Work out the finished part from the listing and answer in its coordinate system (mm). Face numbers are marked on the shaded views. A direction names the side the tool comes from. Round coordinates to 2 decimals unless told otherwise and drop trailing zeros. Loops run counter-clockwise (first coordinate to the right, second up) from the corner with the lowest first, then second, coordinate; pieces in that order, holes last. Notation, with made-up numbers: M -15.75,9.25 L 2.25,9.25 A25 ccw 2.25,25.25 Z; hole C 35.5,28 d8. An arc over 180 degrees is marked long. One line per item, written item: value.
Autodesk Inventor part; units mm, degrees
ref_plane "YZ Plane" through (0, 0, 0) normal (1, 0, 0) x (0, 1, 0)
ref_plane "XZ Plane" through (0, 0, 0) normal (0, 1, 0) x (-1, 0, 0)
ref_plane "XY Plane" through (0, 0, 0) normal (0, 0, 1) x (1, 0, 0)
sketch "Sketch1" plane through (0, 0, 0) normal (0, 1, 0) x (-1, 0, 0)
  line L0 (0, 0) -> (-127, 0)
  line L1 (-127, 0) -> (-127, -124.46)
  line L2 (-127, -124.46) -> (0, -124.46)
  line L3 (0, -124.46) -> (0, 0)
  dimension "d0" = 127
  dimension "d1" = 124.46
extrude "Extrusion1" add sketch "Sketch1" along normal blind 6.35
sketch "Sketch2" plane through (0, 0, 0) normal (0, 0, 1) x (1, 0, 0)
  line L0 (0, 6.35) -> (127, 6.35) construction
  line L1 (0, 6.35) -> (2.921, 6.35) construction
  line L2 (0, 0) -> (127, 0) construction
  line L3 (127, 3.429) -> (127, 2.921) construction
  line L4 (0, 6.35) -> (0, 4.191) construction
  line L5 (0, 0) -> (0, 6.35) construction
  line L6 (0, 6.35) -> (2.159, 6.35) construction
  line L7 (0, 0) -> (0, 2.159) construction
  line L8 (0, 4.191) -> (0, 2.159)
  line L9 (0, 2.159) -> (127, 2.159)
  line L10 (127, 2.159) -> (127, 4.191)
  line L11 (127, 4.191) -> (0, 4.191)
  dimension "d9" = 2.159
  dimension "d10" = 90
  dimension "d11" = 2.159
extrude "Extrusion2" add sketch "Sketch2" along normal blind 12.7
properties part number "False_Bottom_3"
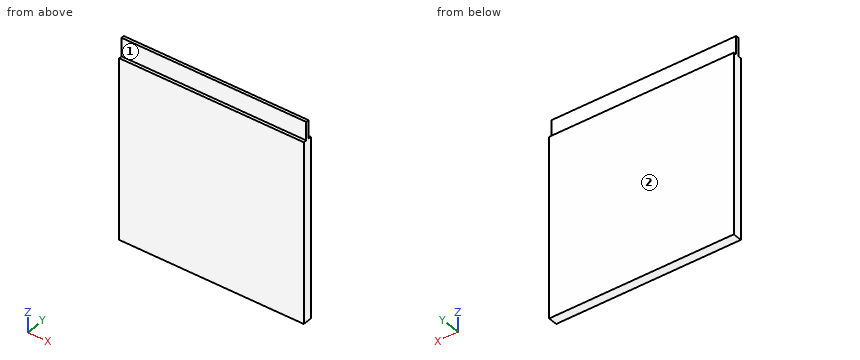
1) Each of these flat-tipped pins is pushed along its axis until it touches: pin 1 (6.5 mm diameter, centred on x = 40, z = 8, fed in from +Y); pin 2 (2.5 mm diameter, centred on x = 55.5, y = 0.5, fed in from +Z); pin 3 (4 mm diameter, centred on x = 86.5, z = 6, fed in from -Y). Where does it stop, or does it pass through?
Check values:
pin 1: y = 4.19
pin 2: z = 0
pin 3: y = 2.16
2) Find the intervals of material crossed by probe 1 along Z at (x, y) = (12, 1.75); probe 2 along Y at (x, z) = (107, 0.5), in increasing order. Write a range as from..to.
Check values:
probe 1: -124.46..0
probe 2: 2.16..4.19
3) Find section A-A (x = 39.5). Give the vertices of the cut face in (y, z).
Check values:
outline: M 0,-124.46 L 6.35,-124.46 L 6.35,0 L 4.19,0 L 4.19,12.7 L 2.16,12.7 L 2.16,0 L 0,0 Z
4) For the marked faces 1 and 2, determine the directions among +Z, -Z, +X, -X, +Y, -Y from which every point of the face is accessible in a straight line to the end or side of a thin tool.
Check values:
face 1: +Z, +X, -X, -Y
face 2: +Z, -Z, +X, -X, +Y
